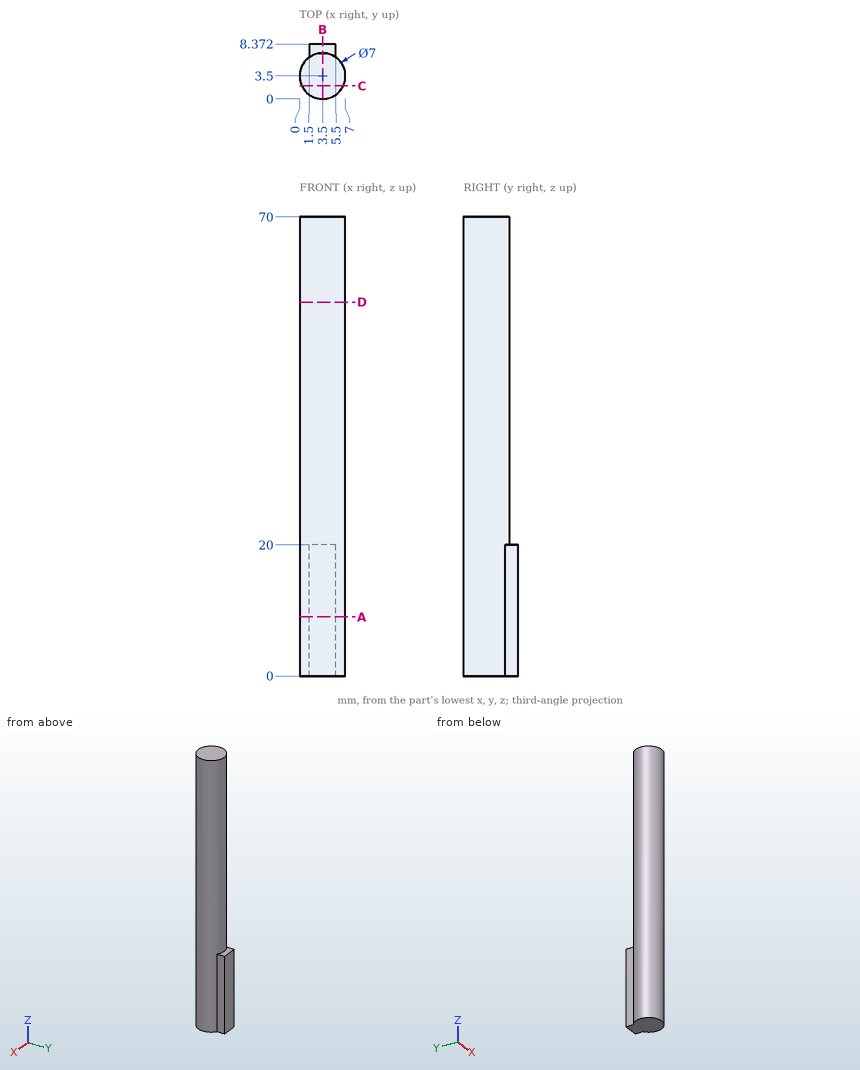
Could you check a few things on this drawing? It's one solid part, dimensions in mm from its lowest x, y, z. Coordinates: 2 decimals unless noted, no trailing zeros. Order: outer loops, then holes, each group sorted by start corner. A loop starts at its lowest first (then second) coordinate and runs counter-clockwise, first axis right, second up.
1) Imagine slicing it at D-D on z = 57. List the corners of the cut face in (x, y) for me, and give its area (3 significant figures).
2) I need wall thicknesses on line 1 (Z direction, x = 2.25, y = 7); line 2 (Y direction, x = 3.25, z = 54). Which ranges of each line are inside material? Lowest first, please.
3) Imagine slicing it at B-B on x = 3.5. List the corners of the cut face in (y, z) for me.
4) Imagine slicing it at C-C on y = 2. List the corners of the cut face in (x, z) for me, and give its area (3 significant figures).
5) Imagine slicing it at A-A on z = 9. List the corners of the cut face in (x, y) for me.
6) Will these pins go through, and if not, where does the flat tip stop? pin 1 (5 mm diameter, centred on y = 2, z = 42, fed in from +X); pin 2 (3 mm diameter, centred on y = 1, z = 43, fed in from +X); pin 3 (2 mm diameter, centred on y = 7.5, z = 8, fed in from -X); pin 4 (1 mm diameter, centred on y = 7.5, z = 13.5, fed in from +X).
Response values:
1. outline: circle Ø7 at (3.5, 3.5)
1. area: 38.5 mm2
2. line 1: z = 0 to 20
2. line 2: y = 0.01 to 6.99
3. outline: (0, 0) - (8.37, 0) - (8.37, 20) - (7, 20) - (7, 70) - (0, 70) - close
4. outline: (0.34, 0) - (6.66, 0) - (6.66, 70) - (0.34, 70) - close
4. area: 443 mm2
5. outline: (1.5, 6.37) arc R3.5 ccw (long way) to (5.5, 6.37) - (5.5, 8.37) - (1.5, 8.37) - close
6. pin 1: stops at x = 7
6. pin 2: stops at x = 6.85
6. pin 3: stops at x = 1.5
6. pin 4: stops at x = 5.5
